```python
from build123d import *

# Parameters (mm, degrees)
SZKIC1_W                    = 350
SZKIC1_H                    = 600
DODANIE_WYCI_GNI_CIE1_DEPTH = 150
WYTNIJ_WYCI_GNI_CIE1_START  = -2.5
SZKIC2_W                    = 300
SZKIC2_H                    = 250
WYTNIJ_WYCI_GNI_CIE1_DEPTH  = 100
SZKIC3_R                    = 17.5
DODANIE_WYCI_GNI_CIE2_DEPTH = 5


with BuildPart() as part:
    # Szkic1 → Dodanie-wyciągnięcie1 (new body)
    with BuildSketch(Plane.XY):
        with Locations((175, 300)):
            Rectangle(SZKIC1_W, SZKIC1_H)
    extrude(amount=DODANIE_WYCI_GNI_CIE1_DEPTH)

    # Szkic2 → Wytnij-wyciągnięcie1 (cut)
    with BuildSketch(Plane(origin=(0, 0, 0), x_dir=(-1, 0, 0), z_dir=(0, 0, -1)).offset(WYTNIJ_WYCI_GNI_CIE1_START)):
        with Locations((-175, 150)):
            Rectangle(SZKIC2_W, SZKIC2_H)
    extrude(amount=-WYTNIJ_WYCI_GNI_CIE1_DEPTH, mode=Mode.SUBTRACT)

    # Szkic3 → Dodanie-wyciągnięcie2 (add)
    with BuildSketch(Plane(origin=(350, 0, 0), x_dir=(0, 0, -1), z_dir=(1, 0, 0))):
        with Locations((-75, 17.5)):
            Circle(SZKIC3_R)
    dodanie_wyci_gni_cie2 = extrude(amount=DODANIE_WYCI_GNI_CIE2_DEPTH)

    # Lustro1: Dodanie-wyciągnięcie2 across plane
    add(dodanie_wyci_gni_cie2.mirror(Plane.ZY.offset(-175)))


solid = part.part
```
Could you check a few things on this model? Use its own coordinates, in mm. A direction names the side the tool comes from. Round coordinates to 2 decimals unless told otherwise and drop trailing zeros. Loops run counter-clockwise (first coordinate to the right, second up) from the corner with the lowest first, then second, coordinate; pieces in that order, holes last. Notation, with made-up numbers: M 42,65.5 L 96,65.5 A18 ccw 96,87.5 Z; hole C 32,78 d7. An arc over 180 degrees is marked long. Write item = value, one per line.
1. I want a section at B-B, the plane x = 37. Write out the boundary of the cut face in (y, z).
Results below:
outline = M 0,0 L 600,0 L 600,150 L 0,150 Z; hole M 25,2.5 L 275,2.5 L 275,102.5 L 25,102.5 Z
2. Will this pin go through, and if not, where does the flat tip stop? P1, Ø8, axis at y = 74.5, z = 82.5, coming from the +X side.
Results below:
P1 = 350
3. I need wall thicknesses on probe 1 along X at (y, z) = (120, 90.5); probe 2 along Z at (x, y) = (199, 156); probe 3 along Y at (x, z) = (314, 47). Which ranges of each line are inside material? Lowest first, please.
Results below:
probe_1 = 0 to 25, 325 to 350
probe_2 = 0 to 2.5, 102.5 to 150
probe_3 = 0 to 25, 275 to 600
4. I want a section at D-D, the plane z = 131. Write out the boundary of the cut face in (x, y).
Results below:
outline = M 0,0 L 350,0 L 350,600 L 0,600 Z
5. Thinking about a two-plate mould opening in Z: for faces 4 (the face through (355, 18, 75)), 5 (the face through (173, 304, 150)), 6 (the face through (177, 25, 52)), which applies, +Z half, -Z half, draft (parallel to the pull), parting line (faces both ways), or undercut?
Results below:
face_4 = draft
face_5 = +Z half
face_6 = undercut
6. Which directions (+Z, -Z, +X, -X, +Y, -Y) give clear straight access to the entire face, cutting with the end or side of a thin tool? Please do faces 1 (the face through (-2.465, 32.256, 65.592)), 2 (the face through (352.465, 32.256, 65.592)), 3 (the face through (177, 152, 2.5)).
Results below:
face_1 = -X
face_2 = +X
face_3 = none
7. I want a section at A-A, the plane y = 252.5. Write out the boundary of the cut face in (x, z), and give its area (3 significant figures).
Results below:
outline = M 0,0 L 350,0 L 350,150 L 0,150 Z; hole M 25,2.5 L 325,2.5 L 325,102.5 L 25,102.5 Z
area = 22,500 mm²
8. I want a section at C-C, the plane y = 17.5. Write out the boundary of the cut face in (x, z).
Results below:
outline = M -5,57.5 L 0,57.5 L 0,0 L 350,0 L 350,57.5 L 355,57.5 L 355,92.5 L 350,92.5 L 350,150 L 0,150 L 0,92.5 L -5,92.5 Z
